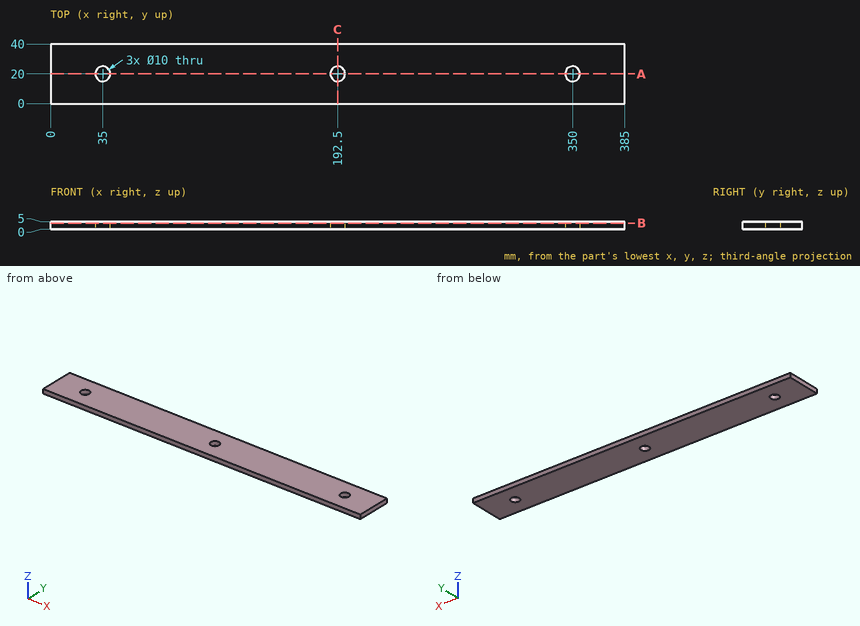
Answer from the drawing. Dimensions are ordinates in mm from the lowest x, y and z of the part. Round coordinates to 2 decimals unless told otherwise and drop trailing zeros. Loops run counter-clockwise (first coordinate to the right, second up) from the corner with the lowest first, then second, coordinate; pieces in that order, holes last.
1) A cutting plane is placed at A-A on y = 20. Determine the outline of the cut face in (x, z), plus the area to 4 significant figures.
Outcome:
outline: (0, 0) - (30, 0) - (30, 5) - (0, 5) - close; (40, 0) - (187.5, 0) - (187.5, 5) - (40, 5) - close; (197.5, 0) - (345, 0) - (345, 5) - (197.5, 5) - close; (355, 0) - (385, 0) - (385, 5) - (355, 5) - close
area: 1,775 mm2
2) A cutting plane is placed at C-C on x = 192.5. Determine the outline of the cut face in (y, z), plus the area to 3 significant figures.
Outcome:
outline: (0, 0) - (15, 0) - (15, 5) - (0, 5) - close; (25, 0) - (40, 0) - (40, 5) - (25, 5) - close
area: 150 mm2
3) A cutting plane is placed at B-B on z = 4.05. Determine the outline of the cut face in (x, y).
Outcome:
outline: (0, 0) - (385, 0) - (385, 40) - (0, 40) - close; hole circle Ø10 at (35, 20); hole circle Ø10 at (192.5, 20); hole circle Ø10 at (350, 20)
4) Consider line 1 (Y direction, x = 350, z = 3.85); line 2 (X direction, y = 22, z = 3.3); line 3 (X direction, y = 17, z = 0.25). Determine where each line is inside the solid, lowest interval first.
Outcome:
line 1: y = 0 to 15, 25 to 40
line 2: x = 0 to 30.42, 39.58 to 187.92, 197.08 to 345.42, 354.58 to 385
line 3: x = 0 to 31, 39 to 188.5, 196.5 to 346, 354 to 385
